Model file for the job. Use its own axes, mm. Face numbers are marked on the shaded views. A direction names the side the tool comes from. Coordinates: 2 decimals unless noted, no trailing zeros. Write each loop counter-clockwise with the first axis right and the second up, starting at its lowest first coordinate (ties: lowest second). Pieces come first, ordered by that corner, then holes.
Q1. Pin check, flat tips, straight feed: P1, Ø10, axis at y = 9, z = 31.5, coming from the +X side; P2, Ø6, axis at y = 5, z = 8.5, coming from the +X side; P3, Ø4, axis at x = -8.5, y = -5, coming from the -Z side; P4, Ø8, axis at y = -1, z = 26, coming from the -X side. Stop position of each tip, or through.
Q2. Which spindle directions (+Z, -Z, +X, -X, +Y, -Y) get a long thin tool onto all of the face, cutting with end or side? Do the marked faces 1 and 2. Say none if no direction does.
Q3. Band-saw the part on A-A, the plane z = 47. Write the cut outline in (x, y), plus the area to 3 significant figures.
Q4. Drill centre lines: probe 1 along Z at (x, y) = (-5.25, 9); probe 2 along X at (y, z) = (-0.5, 30.5); probe 3 along Y at (x, z) = (-0.25, 37.5). Where is each one in solid material? Low to high.
Autodesk Inventor part; units mm, degrees
ref_plane "YZ Plane" through (0, 0, 0) normal (1, 0, 0) x (0, 1, 0)
ref_plane "XZ Plane" through (0, 0, 0) normal (0, 1, 0) x (-1, 0, 0)
ref_plane "XY Plane" through (0, 0, 0) normal (0, 0, 1) x (1, 0, 0)
sketch "Skizze1" plane through (0, 0, 0) normal (0, 0, 1) x (1, 0, 0)
  circle A0 centre (0, 0) radius 13.13
  circle A1 centre (0, 0) radius 4
  dimension "d0" = 26.26
  dimension "d3" = 8
extrude "Extrusion1" add sketch "Skizze1" along normal blind 50 contours A0 | A1
extrude "Extrusion2" add sketch "Skizze1" against normal blind 1 contours A1
fillet "Rundung1" radius 1 2 edges at (-13.13, 0, 0) (-13.13, 0, 50)
properties part number "LG INR18650MJ1"
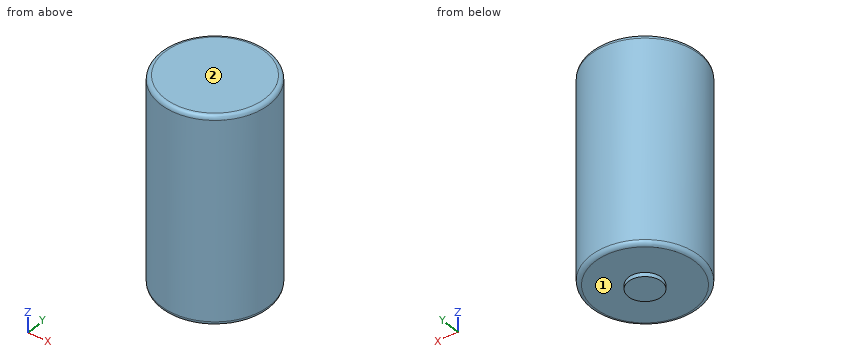
Answer sheet:
1. P1: stops at x = 12.51
1. P2: stops at x = 12.98
1. P3: stops at z = 0
1. P4: stops at x = -13.13
2. face 1: -Z
2. face 2: +Z, +X, -X, +Y, -Y
3. outline: circle Ø26.26 at (0, 0)
3. area: 542 mm2
4. probe 1: z = 0 to 50
4. probe 2: x = -13.12 to 13.12
4. probe 3: y = -13.13 to 13.13
